from build123d import *

# Parameters (mm, degrees)
CROQUIS1_W              = 28.85
CROQUIS1_H              = 31.5
SALIENTE_EXTRUIR1_DEPTH = 17.6
CROQUIS3_W              = 3.368460879
CROQUIS3_H              = 31.5
CROQUIS3_W_2            = 4.327912621
CROQUIS3_W_3            = 3.609366076
CROQUIS3_W_4            = 3.655054254
CROQUIS3_W_5            = 2.924043404
SALIENTE_EXTRUIR2_DEPTH = 9.73
CROQUIS4_W              = 31.5
CROQUIS4_H              = 6.64
SALIENTE_EXTRUIR3_DEPTH = 5.59
CROQUIS5_W              = 31.5
CROQUIS5_H              = 6.64
SALIENTE_EXTRUIR4_DEPTH = 5.59


with BuildPart() as part:
    # Croquis1 → Saliente-Extruir1 (new body)
    with BuildSketch(Plane(origin=(0, 0, 0), x_dir=(1, 0, 0), z_dir=(0, 1, 0))):
        with Locations((14.425, 15.75)):
            Rectangle(CROQUIS1_W, CROQUIS1_H)
    extrude(amount=SALIENTE_EXTRUIR1_DEPTH)

    # Croquis3 → Saliente-Extruir2 (add)
    with BuildSketch(Plane(origin=(0, 17.6, 0), x_dir=(1, 0, 0), z_dir=(0, 1, 0))):
        with Locations((1.68423044, 15.75)):
            Rectangle(CROQUIS3_W, CROQUIS3_H)
        with Locations((26.68604369, 15.75)):
            Rectangle(CROQUIS3_W_2, CROQUIS3_H)
        with Locations((19.884737293, 15.75)):
            Rectangle(CROQUIS3_W_3, CROQUIS3_H)
        with Locations((13.693989149, 15.75)):
            Rectangle(CROQUIS3_W_4, CROQUIS3_H)
        with Locations((7.663149629, 15.75)):
            Rectangle(CROQUIS3_W_5, CROQUIS3_H)
    extrude(amount=SALIENTE_EXTRUIR2_DEPTH)

    # Croquis4 → Saliente-Extruir3 (add)
    with BuildSketch(Plane.ZY):
        with Locations((-15.75, 12.4)):
            Rectangle(CROQUIS4_W, CROQUIS4_H)
    extrude(amount=SALIENTE_EXTRUIR3_DEPTH)

    # Croquis5 → Saliente-Extruir4 (add)
    with BuildSketch(Plane(origin=(28.85, 0, 0), x_dir=(0, 0, -1), z_dir=(1, 0, 0))):
        with Locations((15.75, 12.4)):
            Rectangle(CROQUIS5_W, CROQUIS5_H)
    extrude(amount=SALIENTE_EXTRUIR4_DEPTH)


solid = part.part
Input: part model. Units: mm. Frame: model coordinates. A direction names the side the tool comes from. Give positions to 0.01 mm unless a question says otherwise; leave off trailing zeros. Loops run counter-clockwise (first coordinate to the right, second up) from the corner with the lowest first, then second, coordinate; pieces in that order, holes last. Notation, with made-up numbers: (49.25, 13) -> (56.25, 13) arc R13 ccw to (56.25, 29) -> close; hole circle Ø5 at (46.25, 42). An arc over 180 degrees is marked (long way). Answer as a JSON object with one key per item and string values. Group by question number.
Item 1: Line query: probe 1 along X at (y, z) = (22, -15); probe 2 along Y at (x, z) = (22, -1.5); probe 3 along Y at (x, z) = (-1.5, -12.5). Output: solid intervals per line, ascending.
Item 2: Reachability of faces 4 (the flat face through (-3, 15.72, -16)), 5 (the flat face through (0, 4, -16)), 6 (the flat face through (10, 17.6, -16)), 7 (the flat face through (27, 27.33, -16)) from +Z, -Z, +X, -X, +Y, -Y: full face, straight path, thin tool, end or side. Return the list, or none.
Item 3: Cut plane B-B, the plane z = -11. Return the cut outline in (x, y).
Item 4: Cut plane A-A, the plane y = 20.5. Return the cut outline in (x, z), and give its area (3 significant figures).
Item 5: Cut plane D-D, the plane y = 6. Return the cut outline in (x, z), and give its area (3 significant figures).
Item 6: Pin query (flat end, axial travel): P1, Ø1.4, axis at x = 4.5, z = -8.5, coming from the +Y side; P2, Ø6, axis at y = 19, z = -8.5, coming from the -X side; P3, Ø1.7, axis at x = 31, z = -18, coming from the -Y side; P4, Ø2, axis at x = 11, z = -16, coming from the +Y side. Return the tip coordinate at first contact, or that it passes through.
Item 7: Cut plane C-C, the plane x = 17. Return the cut outline in (y, z).
Item 8: Pull-direction query (X, two-part tool) for faces 1 (the flat face through (0, 21, -16)), 2 (the flat face through (21.689, 22, -16)), 3 (the flat face through (32, 15.72, -16)); classes: released by +X, released by -X, zero draft, split by the parting line, or undercut.
Checks:
{
 "1": {"probe 1": "x = 0 to 3.37, 6.2 to 9.13, 11.87 to 15.52, 18.08 to 21.69, 24.52 to 28.85", "probe 2": "y = 0 to 17.6", "probe 3": "y = 9.08 to 15.72"},
 "2": {"face 4": "+Z, -Z, -X, +Y", "face 5": "+Z, -Z, -X, -Y", "face 6": "+Z, -Z, +Y", "face 7": "+Z, -Z, +X, -X, +Y"},
 "3": {"outline": "(-5.59, 9.08) -> (0, 9.08) -> (0, 0) -> (28.85, 0) -> (28.85, 9.08) -> (34.44, 9.08) -> (34.44, 15.72) -> (28.85, 15.72) -> (28.85, 27.33) -> (24.52, 27.33) -> (24.52, 17.6) -> (21.69, 17.6) -> (21.69, 27.33) -> (18.08, 27.33) -> (18.08, 17.6) -> (15.52, 17.6) -> (15.52, 27.33) -> (11.87, 27.33) -> (11.87, 17.6) -> (9.13, 17.6) -> (9.13, 27.33) -> (6.2, 27.33) -> (6.2, 17.6) -> (3.37, 17.6) -> (3.37, 27.33) -> (0, 27.33) -> (0, 15.72) -> (-5.59, 15.72) -> close"},
 "4": {"outline": "(0, -31.5) -> (3.37, -31.5) -> (3.37, 0) -> (0, 0) -> close; (6.2, -31.5) -> (9.13, -31.5) -> (9.13, 0) -> (6.2, 0) -> close; (11.87, -31.5) -> (15.52, -31.5) -> (15.52, 0) -> (11.87, 0) -> close; (18.08, -31.5) -> (21.69, -31.5) -> (21.69, 0) -> (18.08, 0) -> close; (24.52, -31.5) -> (28.85, -31.5) -> (28.85, 0) -> (24.52, 0) -> close", "area": "563 mm²"},
 "5": {"outline": "(0, -31.5) -> (28.85, -31.5) -> (28.85, 0) -> (0, 0) -> close", "area": "909 mm²"},
 "6": {"P1": "stops at y = 17.6", "P2": "stops at x = 0", "P3": "stops at y = 9.08", "P4": "stops at y = 27.33"},
 "7": {"outline": "(0, -31.5) -> (17.6, -31.5) -> (17.6, 0) -> (0, 0) -> close"},
 "8": {"face 1": "released by -X", "face 2": "undercut", "face 3": "zero draft"}
}
